```python
from build123d import *

# Parameters (mm, degrees)
SKETCH_1_R      = 0.8
EXTRUDE_1_DEPTH = 31
SKETCH_2_R      = 1.5
EXTRUDE_2_DEPTH = 30


with BuildPart() as part:
    # 草图1 → 凸台-拉伸1 (new, symmetric)
    with BuildSketch(Plane(origin=(0, 0, 0), x_dir=(1, 0, 0), z_dir=(0, 1, 0))):
        with Locations(Location((0, 0, 0), (0, 0, 270))):
            Circle(SKETCH_1_R)
    extrude(amount=EXTRUDE_1_DEPTH, both=True)

    # 草图2 → 凸台-拉伸2 (add, symmetric)
    with BuildSketch(Plane(origin=(0, 0, 0), x_dir=(1, 0, 0), z_dir=(0, 1, 0))):
        with Locations(Location((0, 0, 0), (0, 0, 270))):
            Circle(SKETCH_2_R)
    extrude(amount=EXTRUDE_2_DEPTH, both=True)


solid = part.part
```
CAD build for the part. Positions are in the model's coordinates, mm. A direction names the side the tool comes from. Give positions to 0.01 mm unless a question says otherwise; leave off trailing zeros. Loops run counter-clockwise (first coordinate to the right, second up) from the corner with the lowest first, then second, coordinate; pieces in that order, holes last. Notation, with made-up numbers: (50, 75) - (57, 75) arc R23 ccw to (57, 87) - close; hole circle Ø1 at (-0.75, 15). An arc over 180 degrees is marked (long way). Put each result on its own line as item: value.
Q1. Slice it at B-B (z = 0). Give the cut face in (x, y).
Filled in:
outline: (-1.5, -30) - (-0.8, -30) - (-0.8, -31) - (0.8, -31) - (0.8, -30) - (1.5, -30) - (1.5, 30) - (0.8, 30) - (0.8, 31) - (-0.8, 31) - (-0.8, 30) - (-1.5, 30) - close
Q2. Slice it at A-A (x = 0). Give the cut face in (y, z).
Filled in:
outline: (-31, -0.8) - (-30, -0.8) - (-30, -1.5) - (30, -1.5) - (30, -0.8) - (31, -0.8) - (31, 0.8) - (30, 0.8) - (30, 1.5) - (-30, 1.5) - (-30, 0.8) - (-31, 0.8) - close
Q3. Probe line 1 along Y through (x, z) = (0.4, -1.3); line 2 along X through (y, z) = (-26.5, -0.2); line 3 along X through (y, z) = (11, 0.85). List the from-to ranges inside material, lowest first.
Filled in:
line 1: y = -30 to 30
line 2: x = -1.49 to 1.49
line 3: x = -1.24 to 1.24
Q4. Tool access for faces 1 (the face through (-0.49, -30.49, -0.63)), 2 (the face through (0, -31, 0)), 3 (the face through (-0.49, 30.51, -0.63)): list every direction of +Z, -Z, +X, -X, +Y, -Y with a clear straight run to the whole face (end or side of a thin tool).
Filled in:
face 1: -Y
face 2: +Z, -Z, +X, -X, -Y
face 3: +Y
Q5. Slice it at C-C (y = 7). Give the cut face in (x, z).
Filled in:
outline: circle Ø3 at (0, 0)
